The model under review builds one solid part; all positions refer to its coordinate system, in mm. A direction names the side the tool comes from. Round coordinates to 2 decimals unless told otherwise and drop trailing zeros. Order: outer loops, then holes, each group sorted by start corner. A loop starts at its lowest first (then second) coordinate and runs counter-clockwise, first axis right, second up. Notation, with made-up numbers: (40.5, 88) - (48.5, 88) arc R23 cw to (48.5, 102) - close; hole circle Ø6 at (-24.5, -4). An arc over 180 degrees is marked (long way). One line per question, with ' | ' between items. Start each with the question number.
Item 1: Add section D-D on y = 81. State the section outline as (x, z) points, and give its area (3 significant figures).
Item 2: For L1, parallel to X at y = 13.5, z = 0; L2, parallel to X at y = 75, z = 0; L3, parallel to Y at x = 165, z = -46, list the stretches that pass through material, from the lowest coordinate up. Write a range as [from, to].
Item 3: Add section A-A on x = 250. State the section outline as (y, z) points.
Item 4: Add section B-B on z = 0. State the section outline as (x, y) points.
Item 5: Draft analysis for pull direction X (two halves, no side actions). For faces 1 (the face through (264.872, 12.675, -1.953)), 2 (the face through (290, 45, 50)), 3 (the face through (23.26, 57.39, 58.01)), 4 (the face through (97, 0, -1)), state which applies: +X half, -X half, draft (parallel to the pull), parting line (faces both ways), or undercut.
Item 6: Insertion check: pin 1 Ø6 at (y, z) = (68, 57.5) entering from +X; pin 2 Ø12 at (x, y) = (83.5, 26) entering from +Z; pin 3 Ø9 at (x, y) = (216.5, 37.5) entering from -Z; pin 4 Ø18 at (x, z) = (250, 0) entering from -Y. Each pin has a flat end and moves straight along its axis. Give the tip position at first contact, or say it passes through.
Item 7: Tool access review of faces 5 (the face through (191, 27, -62.5)), 6 (the face through (125, 40, 1)), 7 (the face through (187, 27, 62.5)): name each direction out of +Z, -Z, +X, -X, +Y, -Y from which nothing blocks a thin tool from reaching the whole face with its end or side.
Item 8: Add section C-C on x = 0. State the section outline as (y, z) points, and give its area (4 significant figures).
from build123d import *

# Parameters (mm, degrees)
SKETCH1_R           = 62.5
BOSS_EXTRUDE1_DEPTH = 25
SKETCH1_3_R         = 62.5
BOSS_EXTRUDE2_DEPTH = 55
SKETCH1_4_R         = 100
SKETCH1_4_R_2       = 62.5
BOSS_EXTRUDE3_DEPTH = 95
SKETCH3_R           = 15
CUT_EXTRUDE1_DEPTH  = 324.882694814
CHAMFER1_SIZE       = 20


with BuildPart() as part:
    # Sketch1 → Boss-Extrude1 (new body)
    with BuildSketch(Plane(origin=(0, 0, 0), x_dir=(1, 0, 0), z_dir=(0, 1, 0))):
        with BuildLine():
            Line((300, 62.5), (78.06247498, 62.5))
            ThreePointArc((78.06247498, 62.5), (-100, 0), (78.06247498, -62.5))
            Line((78.06247498, -62.5), (300, -62.5))
            Line((300, -62.5), (300, 62.5))
        make_face()
        with Locations(Location((0, 0, 0), (0, 0, 270))):
            Circle(SKETCH1_R, mode=Mode.SUBTRACT)
    extrude(amount=BOSS_EXTRUDE1_DEPTH)

    # Sketch1_3 → Boss-Extrude2 (add)
    with BuildSketch(Plane(origin=(0, 0, 0), x_dir=(1, 0, 0), z_dir=(0, 1, 0))):
        with BuildLine():
            Line((300, 62.5), (78.06247498, 62.5))
            ThreePointArc((78.06247498, 62.5), (-100, 0), (78.06247498, -62.5))
            Line((78.06247498, -62.5), (300, -62.5))
            Line((300, -62.5), (300, -37.5))
            Line((300, -37.5), (125, -37.5))
            Line((125, -37.5), (125, 37.5))
            Line((125, 37.5), (300, 37.5))
            Line((300, 37.5), (300, 62.5))
        make_face()
        Circle(SKETCH1_3_R, mode=Mode.SUBTRACT)
    extrude(amount=BOSS_EXTRUDE2_DEPTH)

    # Sketch1_4 → Boss-Extrude3 (add)
    with BuildSketch(Plane(origin=(0, 0, 0), x_dir=(1, 0, 0), z_dir=(0, 1, 0))):
        with Locations(Location((0, 0, 0), (0, 0, 38.682187453))):
            Circle(SKETCH1_4_R)
        with Locations(Location((0, 0, 0), (0, 0, 270))):
            Circle(SKETCH1_4_R_2, mode=Mode.SUBTRACT)
    extrude(amount=BOSS_EXTRUDE3_DEPTH)

    # Sketch3 → Cut-Extrude1 (cut, through all)
    with BuildSketch(Plane(origin=(0, 25, 0), x_dir=(1, 0, 0), z_dir=(0, 1, 0))):
        with Locations(Location((250, 0, 0), (0, 0, 270))):
            Circle(SKETCH3_R)
        with Locations(Location((185, 0, 0), (0, 0, 270))):
            Circle(SKETCH3_R)
    extrude(amount=-CUT_EXTRUDE1_DEPTH, mode=Mode.SUBTRACT)

    # Chamfer1
    chamfer1_edges = [part.edges().sort_by_distance(p)[0] for p in [
        (300, 55, 50),
        (300, 55, -50),
    ]]
    chamfer(chamfer1_edges, length=CHAMFER1_SIZE)


solid = part.part
Determined:
1) outline: circle Ø200 at (0, 0); hole circle Ø125 at (0, 0) | area: 19,100 mm2
2) L1: [-100, -62.5], [62.5, 170], [200, 235], [265, 300] | L2: [-100, -62.5], [62.5, 100] | L3: [0, 55]
3) outline: (0, -62.5) - (55, -62.5) - (55, -37.5) - (25, -37.5) - (25, -15) - (0, -15) - close; (0, 15) - (25, 15) - (25, 37.5) - (55, 37.5) - (55, 62.5) - (0, 62.5) - close
4) outline: (-100, 0) - (-62.5, 0) - (-62.5, 95) - (-100, 95) - close; (62.5, 0) - (170, 0) - (170, 25) - (125, 25) - (125, 55) - (100, 55) - (100, 95) - (62.5, 95) - close; (200, 0) - (235, 0) - (235, 25) - (200, 25) - close; (265, 0) - (300, 0) - (300, 25) - (265, 25) - close
5) face 1: undercut | face 2: +X half | face 3: undercut | face 4: draft
6) pin 1: x = 83.84 | pin 2: z = 63.2 | pin 3: z = -62.5 | pin 4: through
7) face 5: -Z, +X, +Y, -Y | face 6: +X, +Y | face 7: +Z, +X, +Y, -Y
8) outline: (0, -100) - (95, -100) - (95, -62.5) - (0, -62.5) - close; (0, 62.5) - (95, 62.5) - (95, 100) - (0, 100) - close | area: 7,125 mm2
